from build123d import *

# Parameters (mm, degrees)
SKETCH7_W                = 95
SKETCH7_H                = 4
BOSS_EXTRUDE4_DEPTH      = 47.5
BOSS_EXTRUDE4_DEPTH_BACK = 47.5
SKETCH8_W                = 105
SKETCH8_H                = 4
BOSS_EXTRUDE5_DEPTH      = 52.5
BOSS_EXTRUDE5_DEPTH_BACK = 52.5
SKETCH9_W                = 115
SKETCH9_H                = 4
BOSS_EXTRUDE6_DEPTH      = 57.5
BOSS_EXTRUDE6_DEPTH_BACK = 57.5
SKETCH10_W               = 85
SKETCH10_H               = 85
CUT_EXTRUDE1_DEPTH       = 8
CUT_EXTRUDE1_DEPTH_BACK  = 3.5
SKETCH12_RX              = 7
SKETCH12_RY              = 5
CUT_EXTRUDE2_DEPTH       = 2
SKETCH13_W               = 10
SKETCH13_H               = 4
CUT_EXTRUDE3_DEPTH       = 29
CUT_EXTRUDE3_DEPTH_BACK  = 1
FILLET4_R                = 3
SKETCH14_W               = 9
SKETCH14_H               = 4.5
CUT_EXTRUDE4_DEPTH       = 2
SKETCH16_W               = 4.5
SKETCH16_H               = 4.5
CUT_EXTRUDE5_DEPTH       = 10


with BuildPart() as part:
    # Sketch7 → Boss-Extrude4 (new body, two sides)
    with BuildSketch(Plane.XY) as boss_extrude4_sk:
        with Locations((0, 2)):
            Rectangle(SKETCH7_W, SKETCH7_H)
    extrude(amount=BOSS_EXTRUDE4_DEPTH)
    extrude(boss_extrude4_sk.sketch, amount=-BOSS_EXTRUDE4_DEPTH_BACK)

    # Sketch8 → Boss-Extrude5 (add, two sides)
    with BuildSketch(Plane.XY) as boss_extrude5_sk:
        with Locations((0, 6)):
            Rectangle(SKETCH8_W, SKETCH8_H)
    extrude(amount=BOSS_EXTRUDE5_DEPTH)
    extrude(boss_extrude5_sk.sketch, amount=-BOSS_EXTRUDE5_DEPTH_BACK)

    # Sketch9 → Boss-Extrude6 (add, two sides)
    with BuildSketch(Plane.XY) as boss_extrude6_sk:
        with Locations((0, 10)):
            Rectangle(SKETCH9_W, SKETCH9_H)
    extrude(amount=BOSS_EXTRUDE6_DEPTH)
    extrude(boss_extrude6_sk.sketch, amount=-BOSS_EXTRUDE6_DEPTH_BACK)

    # Sketch10 → Cut-Extrude1 (cut, two sides)
    with BuildSketch(Plane(origin=(0, 0, 0), x_dir=(1, 0, 0), z_dir=(0, 1, 0))) as cut_extrude1_sk:
        Rectangle(SKETCH10_W, SKETCH10_H)
    extrude(amount=CUT_EXTRUDE1_DEPTH, mode=Mode.SUBTRACT)
    extrude(cut_extrude1_sk.sketch, amount=-CUT_EXTRUDE1_DEPTH_BACK, mode=Mode.SUBTRACT)

    # Sketch12 → Cut-Extrude2 (cut)
    with BuildSketch(Plane(origin=(0, 12, 0), x_dir=(1, 0, 0), z_dir=(0, 1, 0))):
        with Locations((0, 4)):
            Ellipse(SKETCH12_RX, SKETCH12_RY)
    extrude(amount=-CUT_EXTRUDE2_DEPTH, mode=Mode.SUBTRACT)

    # Sketch13 → Cut-Extrude3 (cut, two sides)
    with BuildSketch(Plane(origin=(0, 0, 0), x_dir=(1, 0, 0), z_dir=(0, 1, 0))) as cut_extrude3_sk:
        with Locations((0, 4)):
            Rectangle(SKETCH13_W, SKETCH13_H)
    extrude(amount=CUT_EXTRUDE3_DEPTH, mode=Mode.SUBTRACT)
    extrude(cut_extrude3_sk.sketch, amount=-CUT_EXTRUDE3_DEPTH_BACK, mode=Mode.SUBTRACT)

    # Fillet4
    fillet4_edges = [part.edges().sort_by_distance(p)[0] for p in [
        (-47.5, 2, 47.5),
        (47.5, 2, -47.5),
        (0, 0, 47.5),
        (47.5, 2, 47.5),
        (-52.5, 4, 0),
        (-52.5, 6, -52.5),
        (52.5, 6, -52.5),
        (52.5, 4, 0),
        (0, 4, -52.5),
        (-52.5, 6, 52.5),
        (0, 4, 52.5),
        (52.5, 6, 52.5),
        (-57.5, 8, 0),
        (-57.5, 10, -57.5),
        (57.5, 10, -57.5),
        (57.5, 8, 0),
        (0, 8, -57.5),
        (-57.5, 10, 57.5),
        (0, 8, 57.5),
        (57.5, 10, 57.5),
        (-47.5, 2, -47.5),
        (47.5, 0, 0),
        (-47.5, 0, 0),
        (0, 0, -47.5),
    ]]
    fillet(fillet4_edges, radius=FILLET4_R)

    # Sketch14 → Cut-Extrude4 (cut)
    with BuildSketch(Plane(origin=(0, 12, 0), x_dir=(1, 0, 0), z_dir=(0, 1, 0))):
        with Locations((0, -4.75)):
            Rectangle(SKETCH14_W, SKETCH14_H)
    extrude(amount=-CUT_EXTRUDE4_DEPTH, mode=Mode.SUBTRACT)

    # Sketch16 → Cut-Extrude5 (cut)
    with BuildSketch(Plane(origin=(0, 12, 0), x_dir=(1, 0, 0), z_dir=(0, 1, 0))):
        with Locations((2.25, -4.75)):
            Rectangle(SKETCH16_W, SKETCH16_H)
    extrude(amount=-CUT_EXTRUDE5_DEPTH, mode=Mode.SUBTRACT)


solid = part.part
Part model, mm, in its own coordinate system. A direction names the side the tool comes from. Coordinates: 2 decimals unless noted, no trailing zeros. Loops run counter-clockwise (first coordinate to the right, second up) from the corner with the lowest first, then second, coordinate; pieces in that order, holes last. Notation, with made-up numbers: M -35.75,14.5 L 9.25,14.5 A14 cw 9.25,31.5 Z; hole C 22,31 d4. An arc over 180 degrees is marked long. Use a Markdown table: item, result. Add a question column.
Q1. Which spindle directions (+Z, -Z, +X, -X, +Y, -Y) get a long thin tool onto all of the face, cutting with end or side? Do faces 4 (the cylindrical face through (-51.64, 7.51, 51.6)), 5 (the flat face through (-1, 4, -42.5)), 6 (the flat face through (1, 10, 2.5)), 7 (the cylindrical face through (-51.64, 7.51, -51.6)). Say none if no direction does.
Q2. Cut at C-C (z = 23.5). Write the cut outline in (x, y).
Q3. Cut at A-A (z = 5.5). Write the cut outline in (x, y).
Q4. Cut at D-D (y = 1.5). Write the cut outline in (x, z), and give its area (3 significant figures).
Q5. Pin check, flat tips, straight feed: P1, Ø6.5, axis at y = 3.5, z = 5, coming from the +X side; P2, Ø4, axis at x = 0, y = 4, coming from the -Z side; P3, Ø2, axis at x = -25.5, y = 6.5, coming from the -Z side. Stop position of each tip, or through.
Q6. Mould opens along Z. For faces 1 (the cylindrical face through (51.64, 4.9, 0.69)), 2 (the cylindrical face through (56.6, 11.51, -56.64)), 3 (the flat face through (-2, 10, 5)) say: +Z half, -Z half, draft (parallel to the pull), parting line (faces both ways), or undercut.
Q7. Probe L1, parallel to Y at x = 25.5, z = 2; L2, parallel to X at y = 3.75, z = 39; L3, parallel to Y at x = -42, z = -49. List the from-to ranges inside material, lowest first.
Q8. Cut at B-B (x = -35). Write the cut outline in (y, z), and give its area (3 significant figures).
Worked out:
| question | item | result |
|---|---|---|
| 1 | face 4 | +Z, -X, -Y |
| 1 | face 5 | -Y |
| 1 | face 6 | +Y |
| 1 | face 7 | -Z, -X, -Y |
| 2 | outline | M -57.5,11 A3 ccw -54.5,8 L -52.5,8 L -52.5,7 A3 ccw -49.5,4 L -47.5,4 L -47.5,3 A3 ccw -44.5,0 L -42.5,0 L -42.5,8 L 42.5,8 L 42.5,0 L 44.5,0 A3 ccw 47.5,3 L 47.5,4 L 49.5,4 A3 ccw 52.5,7 L 52.5,8 L 54.5,8 A3 ccw 57.5,11 L 57.5,12 L -57.5,12 Z |
| 3 | outline | M -57.5,11 A3 ccw -54.5,8 L -52.5,8 L -52.5,7 A3 ccw -49.5,4 L -47.5,4 L -47.5,3 A3 ccw -44.5,0 L -42.5,0 L -42.5,8 L 0,8 L 0,10 L -4.5,10 L -4.5,12 L -57.5,12 Z; M 4.5,8 L 42.5,8 L 42.5,0 L 44.5,0 A3 ccw 47.5,3 L 47.5,4 L 49.5,4 A3 ccw 52.5,7 L 52.5,8 L 54.5,8 A3 ccw 57.5,11 L 57.5,12 L 4.5,12 Z |
| 4 | outline | M -47.1,-44.5 A2.6 ccw -44.5,-47.1 L 44.5,-47.1 A2.6 ccw 47.1,-44.5 L 47.1,44.5 A2.6 ccw 44.5,47.1 L -44.5,47.1 A2.6 ccw -47.1,44.5 Z; hole M -42.5,-42.5 L 42.5,-42.5 L 42.5,42.5 L -42.5,42.5 Z |
| 4 | area | 1,640 mm2 |
| 5 | P1 | stops at x = 52.49 |
| 5 | P2 | stops at z = -52.33 |
| 5 | P3 | stops at z = -52.5 |
| 6 | face 1 | draft |
| 6 | face 2 | -Z half |
| 6 | face 3 | undercut |
| 7 | L1 | y = 8 to 12 |
| 7 | L2 | x = -47.5 to -42.5, 42.5 to 47.5 |
| 7 | L3 | y = 4 to 12 |
| 8 | outline | M 0,-44.5 A3 ccw 3,-47.5 L 4,-47.5 L 4,-49.5 A3 ccw 7,-52.5 L 8,-52.5 L 8,-54.5 A3 ccw 11,-57.5 L 12,-57.5 L 12,57.5 L 11,57.5 A3 ccw 8,54.5 L 8,52.5 L 7,52.5 A3 ccw 4,49.5 L 4,47.5 L 3,47.5 A3 ccw 0,44.5 L 0,42.5 L 8,42.5 L 8,-42.5 L 0,-42.5 Z |
| 8 | area | 568 mm2 |
